Answer from the drawing. Dimensions are ordinates in mm from the lowest x, y and z of the part. A direction names the side the tool comes from. Round coordinates to 2 decimals unless told otherwise and drop trailing zeros. Order: outer loops, then holes, each group sorted by start corner. A loop starts at its lowest first (then second) coordinate and runs counter-clockwise, first axis right, second up. Notation, with made-up numbers: (15.25, 55.25) -> (72.25, 55.25) arc R9 cw to (72.25, 63.25) -> close; hole circle Ø9 at (26.5, 30). An arc over 180 degrees is marked (long way). Use a Markdown table: item, result. Add a question column.
1. For the marked faces 1 and 2, determine the directions among +Z, -Z, +X, -X, +Y, -Y from which every point of the face is accessible in a straight line to the end or side of a thin tool.
2. Section C-C, the plane z = 43 is taken. Give the vertices of the cut face in (x, y).
3. Given pin 1 (4 mm diameter, centred on x = 45.5, y = 32.5, fed in from +Z); pin 2 (6.5 mm diameter, centred on y = 25, z = 45.5, fed in from +X); pin 3 (20.5 mm diameter, centred on x = 67.5, y = 26.5, fed in from +Z), each flat-ended and moving along its own axis, determine where each tip first touches the part or whether it passes through.
4. Consider L1, parallel to X at y = 2, z = 15; L2, parallel to Z at x = 52, y = 18; L3, parallel to X at y = 37, z = 44. Determine where each line is inside the solid, lowest interval first. Write a range as [from, to].
5. Section B-B, the plane x = 61 is taken. Give the vertices of the cut face in (y, z).
6. Section A-A, the plane y = 28.5 is taken. Give the vertices of the cut face in (x, z), then the cut area to 3 significant figures.
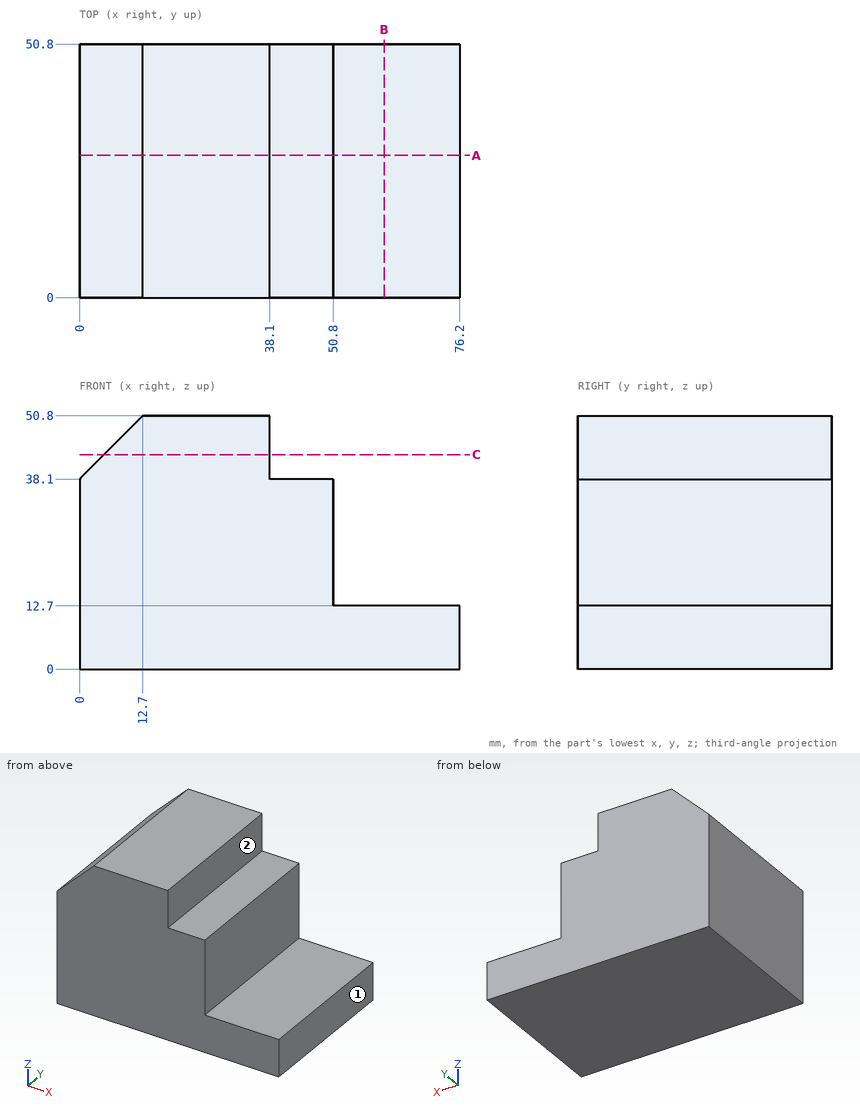
Verdict:
| question | item | result |
|---|---|---|
| 1 | face 1 | +Z, -Z, +X, +Y, -Y |
| 1 | face 2 | +Z, +X, +Y, -Y |
| 2 | outline | (4.9, 0) -> (38.1, 0) -> (38.1, 50.8) -> (4.9, 50.8) -> close |
| 3 | pin 1 | stops at z = 38.1 |
| 3 | pin 2 | stops at x = 38.1 |
| 3 | pin 3 | stops at z = 12.7 |
| 4 | L1 | x = [0, 50.8] |
| 4 | L2 | z = [0, 12.7] |
| 4 | L3 | x = [5.9, 38.1] |
| 5 | outline | (0, 0) -> (50.8, 0) -> (50.8, 12.7) -> (0, 12.7) -> close |
| 6 | outline | (0, 0) -> (76.2, 0) -> (76.2, 12.7) -> (50.8, 12.7) -> (50.8, 38.1) -> (38.1, 38.1) -> (38.1, 50.8) -> (12.7, 50.8) -> (0, 38.1) -> close |
| 6 | area | 2,660 mm2 |
